Design review of the part built by this model. Coordinates are the model's own, in mm. A direction names the side the tool comes from. Coordinates: 2 decimals unless noted, no trailing zeros. Loops run counter-clockwise (first coordinate to the right, second up) from the corner with the lowest first, then second, coordinate; pieces in that order, holes last. Notation, with made-up numbers: M 72.25,25 L 92.25,25 A27 cw 92.25,45 Z; hole C -36,65.5 d3. An arc over 180 degrees is marked long. One line per item, written item: value.
```python
from build123d import *

# Parameters (mm, degrees)
F1_DEPTH      = 15
F2_DEPTH      = 13
F0_R          = 2.75
F3_DEPTH      = 13
F3_DEPTH_BACK = 23.5
F4_T1_DEPTH   = 13


# Not quite as in the source:
# - a fillet or chamfer that OpenCascade refuses, or shapes differently, is made with other operations: its cross-section is extruded or revolved along the edge and cut away or added


with BuildPart() as f1:
    # F0 (on Top) → F1 (new body)
    with BuildSketch(Plane.XY):
        Polygon((2.2306062124, 9.8), (0, 9.8), (-2.2306062124, 9.8), (-5.7, 5.796853322), (-5.7, 2), (-5.7, -2), (-5.7, -9.4), (0, -9.4), (5.7, -9.4), (5.7, 5.796853322), align=None)
        Polygon((-1.5, 8.2), (0, 8.2), (1.5, 8.2), (4.1, 5.2), (4.1, -7.8), (0, -7.8), (-4.1, -7.8), (-4.1, 5.2), align=None, mode=Mode.SUBTRACT)
    extrude(amount=F1_DEPTH)

    # F0 (on Top) → F2 (join)
    with BuildSketch(Plane.XY):
        with BuildLine():
            Line((-5.7, -2), (-5.7, 2))
            Line((-5.7, 2), (-8.0370348177, 2))
            ThreePointArc((-8.0370348177, 2), (-7.6735121825, 1.0292233618), (-7.55, 0))
            ThreePointArc((-7.55, 0), (-7.6735121825, -1.0292233618), (-8.0370348177, -2))
            Line((-8.0370348177, -2), (-5.7, -2))
        make_face()
        with BuildLine():
            ThreePointArc((-7.55, 0), (-7.6735121825, 1.0292233618), (-8.0370348177, 2))
            Line((-8.0370348177, 2), (-8.4, 2))
            Line((-8.4, 2), (-8.4, -2))
            Line((-8.4, -2), (-8.0370348177, -2))
            ThreePointArc((-8.0370348177, -2), (-7.6735121825, -1.0292233618), (-7.55, 0))
        make_face()
    extrude(amount=F2_DEPTH)

    # F0 (on Top) → F3 (join, two sides)
    with BuildSketch(Plane.XY) as f3_sk:
        with BuildLine():
            Line((-8.4, 2), (-8.0370348177, 2))
            ThreePointArc((-8.0370348177, 2), (-16.25, 0), (-8.0370348177, -2))
            Line((-8.0370348177, -2), (-8.4, -2))
            Line((-8.4, -2), (-8.4, 2))
        make_face()
        with Locations((-11.9, 0)):
            Circle(F0_R, mode=Mode.SUBTRACT)
        with BuildLine():
            ThreePointArc((-7.55, 0), (-7.6735121825, 1.0292233618), (-8.0370348177, 2))
            Line((-8.0370348177, 2), (-8.4, 2))
            Line((-8.4, 2), (-8.4, -2))
            Line((-8.4, -2), (-8.0370348177, -2))
            ThreePointArc((-8.0370348177, -2), (-7.6735121825, -1.0292233618), (-7.55, 0))
        make_face()
    extrude(amount=F3_DEPTH)
    extrude(f3_sk.sketch, amount=-F3_DEPTH_BACK)

    # F4: fillet of radius 2 on 4 edges, made by hand

    # F4_s2 → F4_t1 (join)
    with BuildSketch(Plane.XY):
        with BuildLine():
            ThreePointArc((-5.7, -4), (-6.2857864376, -2.5857864376), (-7.7, -2))
            Line((-7.7, -2), (-5.7, -2))
            Line((-5.7, -2), (-5.7, -4))
        make_face()
        with BuildLine():
            ThreePointArc((-5.7, 4), (-6.2857864376, 2.5857864376), (-7.7, 2))
            Line((-7.7, 2), (-5.7, 2))
            Line((-5.7, 2), (-5.7, 4))
        make_face()
        with BuildLine():
            ThreePointArc((-6.9682153332, -2), (-7.8285393886, -2.1944966021), (-8.5215333385, -2.7401574803))
            ThreePointArc((-8.5215333385, -2.7401574803), (-8.2604200708, -2.382426901), (-8.0370348177, -2))
            Line((-8.0370348177, -2), (-6.9682153332, -2))
        make_face()
        with BuildLine():
            ThreePointArc((-6.9682153332, 2), (-7.8285393886, 2.1944966021), (-8.5215333385, 2.7401574803))
            ThreePointArc((-8.5215333385, 2.7401574803), (-8.2604200708, 2.382426901), (-8.0370348177, 2))
            Line((-8.0370348177, 2), (-6.9682153332, 2))
        make_face()
    extrude(amount=F4_T1_DEPTH)


solid = f1.part
```
(1) Mouldability with a two-part tool opening along X and no side actions: class faces 6 (the flat face through (3.99, 7.77, 7.4)), 7 (the flat face through (4.1, -1, 7)), 8 (the flat face through (-4.5, 0.3, 0)) as released by +X, released by -X, zero draft, split by the parting line, or undercut.
Reply:
face 6: released by +X
face 7: undercut
face 8: zero draft
(2) We need section A-A on y = -6.25. State the section outline as (x, z) points, then the cut area to 3 significant figures.
Reply:
outline: M -5.7,0 L -4.1,0 L -4.1,15 L -5.7,15 Z; M 4.1,0 L 5.7,0 L 5.7,15 L 4.1,15 Z
area: 48.0 mm2
(3) Insertion check: pin 1 (9.5 mm diameter, centred on x = -12, y = 0.5, fed in from +Z); pin 2 (1.5 mm diameter, centred on x = -0.5, y = 5.5, fed in from -Z); pin 3 (5 mm diameter, centred on y = -6.5, z = -8, fed in from -X); pin 4 (8 mm diameter, centred on x = -8.5, z = -5.5, fed in from +Y). Each pin has a flat end and moves straight along its axis. Give the tip position at first contact, or say it passes through.
Reply:
pin 1: stops at z = 13
pin 2: passes through
pin 3: stops at x = -13.61
pin 4: stops at y = 4.35
(4) We need section D-D on z = -13. State the section outline as (x, y) points, then the cut area to 3 significant figures.
Reply:
outline: C -11.9,0 d8.7; hole C -11.9,0 d5.5
area: 35.7 mm2
(5) Tool access review of faces 1 (the flat face through (-9.7, 2, 13)), 2 (the cylindrical face through (-7.982, -2.276, 6.409)), 3 (the flat face through (0, 9.8, 7)), 4 (the flat face through (-4.1, -1, 7)), 5 (the cylindrical face through (-6.15, 2.737, 6.409)): name each direction out of +Z, -Z, +X, -X, +Y, -Y from which nothing blocks a thin tool from reaching the whole face with its end or side.
Reply:
face 1: +Z, -X, +Y, -Y
face 2: +Z, -Z, -Y
face 3: +Z, -Z, +X, -X, +Y
face 4: +Z, -Z
face 5: +Z, -Z, +Y
(6) We need section C-C on y = -1.5. State the section outline as (x, z) points, then the cut area to 3 significant figures.
Reply:
outline: M -15.98,-23.5 L -14.2,-23.5 L -14.2,13 L -15.98,13 Z; M -9.6,-23.5 L -7.82,-23.5 L -7.82,0 L -4.1,0 L -4.1,15 L -5.7,15 L -5.7,13 L -9.6,13 Z; M 4.1,0 L 5.7,0 L 5.7,15 L 4.1,15 Z
area: 205 mm2
(7) We need section B-B on x = -11.9. State the section outline as (y, z) points.
Reply:
outline: M -4.35,-23.5 L -2.75,-23.5 L -2.75,13 L -4.35,13 Z; M 2.75,-23.5 L 4.35,-23.5 L 4.35,13 L 2.75,13 Z
(8) To check wall thickness, follow line 1 along X through (y, z) = (-3.75, 7); line 2 along X through (y, z) = (-1, 4.5); line 3 along Y through (x, z) = (-11.9, -1.5). State the ranges of each line that lie inside material, in increasing order. Write a range as [from, to].
Reply:
line 1: x = [-14.1, -9.7], [-5.72, -4.1], [4.1, 5.7]
line 2: x = [-16.13, -14.46], [-9.34, -4.1], [4.1, 5.7]
line 3: y = [-4.35, -2.75], [2.75, 4.35]
